```python
from build123d import *

# Parameters (mm, degrees)
CYLINDER031_R          = 3
CYLINDER031_DEPTH      = 12
CYLINDER031_ROLL_ANGLE = 90
PAD018_DEPTH           = 3
CYLINDER032_R          = 16
CYLINDER032_DEPTH      = 4
CYLINDER032_ROLL_ANGLE = 90


with BuildPart() as cylinder022_holder_axis:
    # Cylinder031 → Cylinder031 (new body)
    with BuildSketch(Plane.XY):
        Circle(CYLINDER031_R)
    extrude(amount=CYLINDER031_DEPTH)


with BuildPart() as cylinder022_holder_axis_1:
    # Cylinder031 roll: moved
    add(cylinder022_holder_axis.part.rotate(Axis((0, 0, 0), (1, 0, 0)), CYLINDER031_ROLL_ANGLE))


with BuildPart() as cylinder022_holder_axis_2:
    # Cylinder031 placement: moved
    add(cylinder022_holder_axis_1.part.moved(Location((-2, -22, 3.5))))


with BuildPart() as pad018:
    # Sketch015 → Pad018 (new body)
    with BuildSketch(Plane.XZ.offset(18)):
        with BuildLine():
            Line((-17.270868, 6), (-2, 8))
            Line((-2, 8), (13.457036, 6.165845))
            ThreePointArc((13.404874, 0.850143), (15.692563, 3.485802), (13.457036, 6.165845))
            Line((13.404874, 0.850143), (-2, -1))
            Line((-2, -1), (-17.581, 1.174724))
            ThreePointArc((-17.270868, 6), (-19.680526, 3.73227), (-17.581, 1.174724))
        make_face()
    extrude(amount=PAD018_DEPTH)


with BuildPart() as camera_rotor:
    # Cylinder032 → Cylinder032 (new body)
    with BuildSketch(Plane.XY):
        Circle(CYLINDER032_R)
    extrude(amount=CYLINDER032_DEPTH)


with BuildPart() as camera_rotor_1:
    # Cylinder032 roll: moved
    add(camera_rotor.part.rotate(Axis((0, 0, 0), (1, 0, 0)), CYLINDER032_ROLL_ANGLE))


with BuildPart() as camera_rotor_2:
    # Cylinder032 placement: moved
    add(camera_rotor_1.part.moved(Location((-2, -18, 3.5))))

    # Cut006: cut Pad018
    add(pad018.part, mode=Mode.SUBTRACT)

    # Fusion004: union Cylinder022-holder-axis
    add(cylinder022_holder_axis_2.part)


solid = camera_rotor_2.part
```
The model under review builds one solid part; all positions refer to its coordinate system, in mm. A direction names the side the tool comes from. Give positions to 0.01 mm unless a question says otherwise; leave off trailing zeros. Write each loop counter-clockwise with the first axis right and the second up, starting at its lowest first coordinate (ties: lowest second). Pieces come first, ordered by that corner, then holes. Notation, with made-up numbers: M 34.25,50 L 86.25,50 A25 ccw 86.25,87 Z; hole C 32.25,-23.75 d4. An arc over 180 degrees is marked long. Write each question's results on one line, items separated by ' | '. Start each with the question number.
1. Insertion check: pin 1 Ø3 at (x, z) = (-6.5, 2.5) entering from +Y; pin 2 Ø4 at (y, z) = (-25.5, -1) entering from +X; pin 3 Ø4 at (x, z) = (-14.5, 0.5) entering from -Y. Each pin has a flat end and moves straight along its axis. Give the tip position at first contact, or say it passes through.
2. For probe 1 along Y at (x, z) = (6, -7); probe 2 along Y at (x, z) = (-13, 2); probe 3 along Z at (x, y) = (-15.5, -20), list the stretches that pass through material, from the lowest coordinate up. Write a range as [from, to].
3. We need section C-C (x = -1.5). Write out the cut boundary in (y, z).
4. Mouldability with a two-part tool opening along X and no side actions: class faces 1 (the cylindrical face through (12.78, -19.97, -2.63)), 2 (the flat face through (-2, -34, 4)), 3 (the flat face through (-9.68, -19.48, 0.07)) as released by +X, released by -X, zero draft, split by the parting line, or undercut.
5. We need section B-B (z = 3.5). Write out the cut boundary in (x, y), and give its area (3 significant figures).
6. We need section D-D (y = -24). Write out the cut boundary in (x, z).
7. For faces 4 (the cylindrical face through (-2.391, -27.916, 6.474)), 5 (the flat face through (-2, -18, -6)), 6 (the flat face through (-9.742, -19.479, 6.986)), list the 3-axis set-ups (+Z, -Z, +X, -X, +Y, -Y) from which the entire face can be reached by the end or side of a thin tool; tool diameter is ignored.
8. We need section A-A (y = -20.5). Write out the cut boundary in (x, z), and give its area (3 significant figures).
Results found:
1) pin 1: stops at y = -21 | pin 2: stops at x = -0.34 | pin 3: stops at y = -22
2) probe 1: y = [-22, -18] | probe 2: y = [-22, -21] | probe 3: z = [-5.09, 0.88], [6.23, 12.09]
3) outline: M -34,0.54 L -22,0.54 L -22,-12.49 L -18,-12.49 L -18,-0.94 L -21,-0.94 L -21,7.94 L -18,7.94 L -18,19.49 L -22,19.49 L -22,6.46 L -34,6.46 Z
4) face 1: split by the parting line | face 2: zero draft | face 3: undercut
5) outline: M -18,-22 L -5,-22 L -5,-34 L 1,-34 L 1,-22 L 14,-22 L 14,-21 L -18,-21 Z | area: 104 mm^2
6) outline: C -2,3.5 d6
7) face 4: -Y | face 5: +Z, -Z, +X, -X, +Y | face 6: +Y
8) outline: M -17.84,1.22 A16 ccw 13.79,0.94 A2.69 cw 13.4,0.85 L -2,-1 L -17.58,1.17 A2.42 cw Z; M -17.81,5.94 A2.42 cw -17.27,6 L -2,8 L 13.46,6.17 A2.69 cw 13.79,6.09 A16 ccw Z | area: 582 mm^2
